For this review, take the finished solid that the model builds, in its own axes (mm). Face numbers are marked on the shaded views. A direction names the side the tool comes from. Coordinates: 2 decimals unless noted, no trailing zeros. Order: outer loops, then holes, each group sorted by start corner. A loop starts at its lowest first (then second) coordinate and runs counter-clockwise, first axis right, second up. Notation, with made-up numbers: (64, 76) -> (83, 76) arc R6 ccw to (83, 83) -> close; hole circle Ø9 at (6.5, 57). An arc over 180 degrees is marked (long way). Answer as a JSON object with one key per item and string values. Group by question number.
1) Add section A-A, the plane y = 5.5. Write out the cut boundary in (x, z).
2) Add section B-B, the plane z = 1. Write out the cut boundary in (x, y).
3) For pin 1 (2 mm diameter, centred on y = 8, z = 6.5, fed in from -X); pin 2 (1.5 mm diameter, centred on y = 6, z = 4, fed in from -X); pin 3 (5 mm diameter, centred on x = 51, z = 5, fed in from +Y), all flat-tipped, find the tip position at first contact; note any pin that passes through.
4) Draft analysis for pull direction Y (two halves, no side actions). For the marked faces 1, 2, 3 and 4, state which applies: +Y half, -Y half, draft (parallel to the pull), parting line (faces both ways), or undercut.
5) Machinability: for the marked faces 5, 6 and 7, which of the approach directions +Z, -Z, +X, -X, +Y, -Y give a long, thin tool a straight path to every point of the face, cutting with its end or side? Answer none if there is none.
6) Wall thickness on L1, parallel to Y at x = 7, z = 3; L2, parallel to X at y = 2.75, z = 4.25; L3, parallel to Y at x = 52, z = 7.5: over which ranges is each line inside the solid? List them lowest first.
7) Add section C-C, the plane z = 5. Write out the cut boundary in (x, y).
8) Add section D-D, the plane x = 36. Write out the cut boundary in (y, z).
from build123d import *

# Parameters (mm, degrees)
SALIENTE_EXTRUIR1_DEPTH = 10
CROQUIS2_R              = 1.5
CORTAR_EXTRUIR1_DEPTH   = 10
CROQUIS3_W              = 15
CROQUIS3_H              = 2.5
CORTAR_EXTRUIR2_DEPTH   = 10
CROQUIS4_R              = 1.5
CORTAR_EXTRUIR3_DEPTH   = 10
CORTAR_EXTRUIR5_DEPTH   = 10
CROQUIS9_R              = 1.5
SALIENTE_EXTRUIR2_DEPTH = 2.5
CROQUIS11_R             = 1.5
CORTAR_EXTRUIR8_DEPTH   = 10
CORTAR_EXTRUIR9_DEPTH   = 58.758116313


with BuildPart() as part:
    # Croquis1 → Saliente-Extruir1 (new body)
    with BuildSketch(Plane.XY):
        Polygon((0, 0), (39.6, 0), (39.6, 2.5), (39.6, 7.5), (39.6, 10), (0, 10), (0, 7.5), (15, 7.5), (15, 2.5), (0, 2.5), align=None)
    extrude(amount=SALIENTE_EXTRUIR1_DEPTH)

    # Croquis2 → Cortar-Extruir1 (cut)
    with BuildSketch(Plane(origin=(0, 10, 0), x_dir=(1, 0, 0), z_dir=(0, 1, 0))):
        with Locations(Location((5, -5, 0), (0, 0, 270))):
            Circle(CROQUIS2_R)
        with BuildLine():
            Line((-4.031911586, 0), (5, 0))
            ThreePointArc((5, 0), (0, -5), (5, -10))
            Line((5, -10), (-4.031911586, -10))
            Line((-4.031911586, -10), (-4.031911586, 0))
        make_face()
    extrude(amount=-CORTAR_EXTRUIR1_DEPTH, mode=Mode.SUBTRACT)

    # Croquis3 → Cortar-Extruir2 (cut)
    with BuildSketch(Plane(origin=(0, 10, 0), x_dir=(1, 0, 0), z_dir=(0, 1, 0))):
        with Locations((32.1, -1.25)):
            Rectangle(CROQUIS3_W, CROQUIS3_H)
        with Locations((32.1, -8.75)):
            Rectangle(CROQUIS3_W, CROQUIS3_H)
    extrude(amount=-CORTAR_EXTRUIR2_DEPTH, mode=Mode.SUBTRACT)

    # Croquis4 → Cortar-Extruir3 (cut)
    with BuildSketch(Plane.XY.offset(7.5)):
        with Locations((34.6, 5)):
            Circle(CROQUIS4_R)
        with BuildLine():
            Line((34.6, 10), (103.004091933, 10))
            Line((103.004091933, 10), (103.004091933, 0))
            Line((103.004091933, 0), (34.6, 0))
            ThreePointArc((34.6, 0), (39.6, 5), (34.6, 10))
        make_face()
    extrude(amount=-CORTAR_EXTRUIR3_DEPTH, mode=Mode.SUBTRACT)

    # Croquis8 → Cortar-Extruir5 (cut)
    with BuildSketch(Plane.XY.offset(7.5)):
        with BuildLine():
            Line((24.6, 0), (34.6, 0))
            ThreePointArc((34.6, 0), (39.6, 5), (34.6, 10))
            Line((34.6, 10), (24.6, 10))
            Line((24.6, 10), (24.6, 0))
        make_face()
    extrude(amount=-CORTAR_EXTRUIR5_DEPTH, mode=Mode.SUBTRACT)

    # Croquis9 → Saliente-Extruir2 (add, symmetric)
    with BuildSketch(Plane(origin=(0, 5, 0), x_dir=(-1, 0, 0), z_dir=(0, -1, 0))):
        with BuildLine():
            Line((-24.6, -10), (-95, -10))
            ThreePointArc((-95, -10), (-100, -5), (-95, 0))
            Line((-95, 0), (-24.6, 0))
            Line((-24.6, 0), (-24.6, -10))
        make_face()
        with Locations(Location((-95, -5, 0), (0, 0, 90))):
            Circle(CROQUIS9_R, mode=Mode.SUBTRACT)
    extrude(amount=SALIENTE_EXTRUIR2_DEPTH, both=True)

    # Croquis11 → Cortar-Extruir8 (cut)
    with BuildSketch(Plane.XZ.offset(-2.5)):
        with Locations(Location((51, 5, 0), (0, 0, 270))):
            Circle(CROQUIS11_R)
        with BuildLine():
            Line((51, 10), (51, 16.019823118))
            Line((51, 16.019823118), (124.451684226, 16.019823118))
            Line((124.451684226, 16.019823118), (123.024656772, -12.837843177))
            Line((123.024656772, -12.837843177), (54.838697363, -9.466010019))
            Line((54.838697363, -9.466010019), (51, 0))
            ThreePointArc((51, 0), (56, 5), (51, 10))
        make_face()
    extrude(amount=-CORTAR_EXTRUIR8_DEPTH, mode=Mode.SUBTRACT)

    # Croquis12 → Cortar-Extruir9 (cut, through all)
    with BuildSketch(Plane.XY.offset(10)):
        Polygon((24.6, 7.5), (17.841989968, 10), (24.6, 10), align=None)
        Polygon((24.6, 2.5), (17.841989968, 0), (24.6, 0), align=None)
    extrude(amount=-CORTAR_EXTRUIR9_DEPTH, mode=Mode.SUBTRACT)


solid = part.part
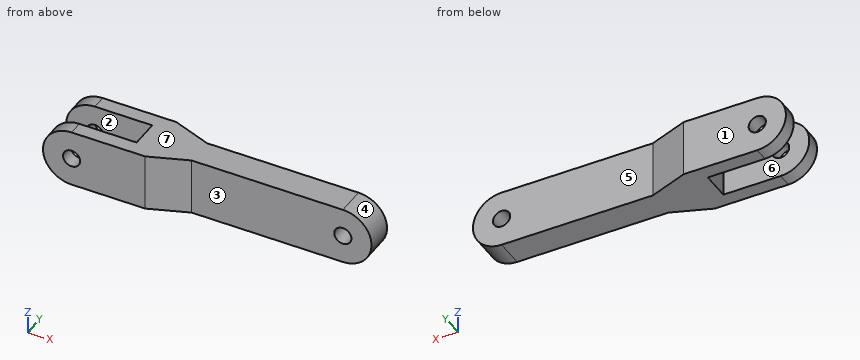
Output values:
{
 "1": {"outline": "(15, 0) -> (51, 0) arc R5 ccw to (51, 10) -> (15, 10) -> close; hole circle Ø3 at (51, 5)"},
 "2": {"outline": "(2, 0) -> (17.84, 0) -> (24.6, 2.5) -> (54, 2.5) -> (54, 7.5) -> (24.6, 7.5) -> (17.84, 10) -> (2, 10) -> (2, 7.5) -> (15, 7.5) -> (15, 2.5) -> (2, 2.5) -> close"},
 "3": {"pin 1": "stops at x = 0.03", "pin 2": "stops at x = 15", "pin 3": "stops at y = 7.5"},
 "4": {"face 1": "+Y half", "face 2": "undercut", "face 3": "-Y half", "face 4": "draft"},
 "5": {"face 5": "+Z, -Z, +X, +Y", "face 6": "+Z, -Z, -X", "face 7": "+Z, +X, -X, +Y, -Y"},
 "6": {"L1": "y = 0 to 2.5, 7.5 to 10", "L2": "x = 15 to 49.7, 52.3 to 55.94", "L3": "y = 2.5 to 7.5"},
 "7": {"outline": "(0, 0) -> (3.5, 0) -> (3.5, 2.5) -> (0, 2.5) -> close; (0, 7.5) -> (3.5, 7.5) -> (3.5, 10) -> (0, 10) -> close; (6.5, 0) -> (17.84, 0) -> (24.6, 2.5) -> (49.5, 2.5) -> (49.5, 7.5) -> (24.6, 7.5) -> (17.84, 10) -> (6.5, 10) -> (6.5, 7.5) -> (15, 7.5) -> (15, 2.5) -> (6.5, 2.5) -> close; (52.5, 2.5) -> (56, 2.5) -> (56, 7.5) -> (52.5, 7.5) -> close"},
 "8": {"outline": "(2.5, 0) -> (7.5, 0) -> (7.5, 10) -> (2.5, 10) -> close"}
}
